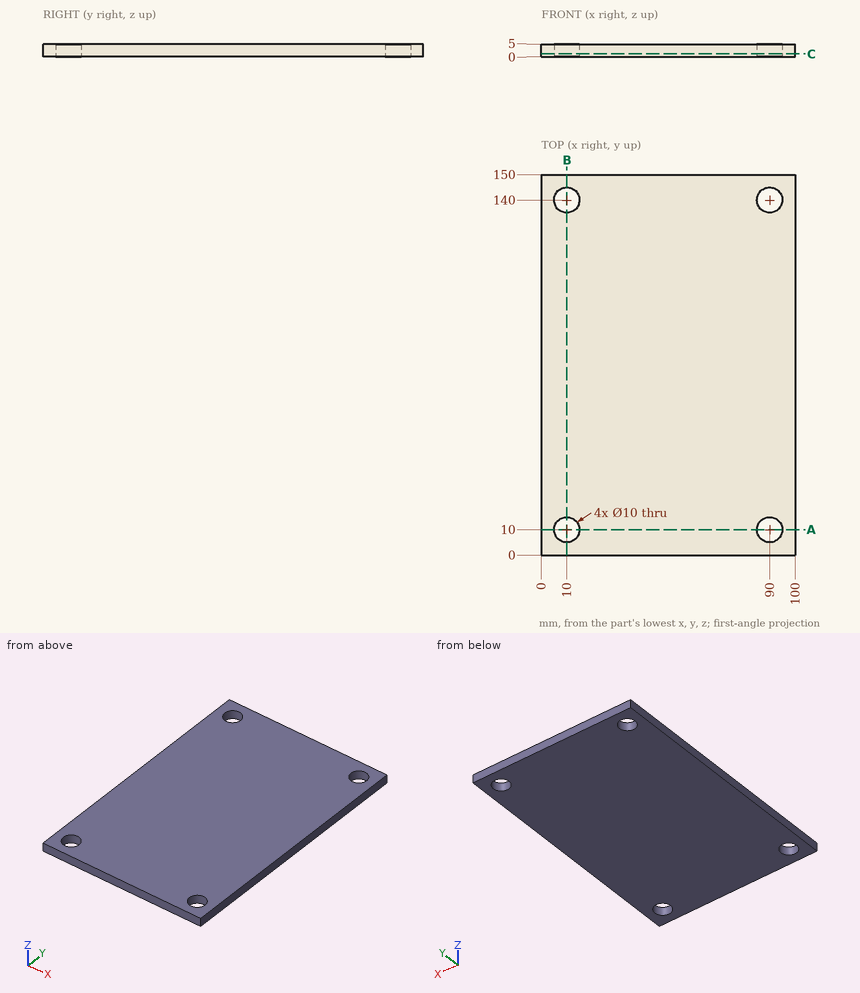
The drawing under review shows one solid part. Ordinate dimensions are in mm from its lowest x, y, z. Give positions to 0.01 mm unless a question says otherwise; leave off trailing zeros. Loops run counter-clockwise (first coordinate to the right, second up) from the corner with the lowest first, then second, coordinate; pieces in that order, holes last. Notation, with made-up numbers: M -0.5,23.25 L 41.5,23.25 A11 cw 41.5,32.25 Z; hole C 12.25,71 d11. An arc over 180 degrees is marked long. Return JSON: item names as keys, results as strings. Group by question number.
Item 1: For probe 1 along Y at (x, z) = (90, 1.4); probe 2 along X at (y, z) = (140, 2.55); probe 3 along X at (y, z) = (143.5, 3), list the stretches that pass through material, from the lowest coordinate up.
Item 2: We need section A-A (y = 10). Give the boundary of the cut face in (x, z).
Item 3: Insertion check: pin 1 Ø8 at (x, y) = (90, 10) entering from +Z. The pin has a flat end and moves straight along its axis. Give the tip position at first contact, or say it passes through.
Item 4: We need section B-B (x = 10). Give the boundary of the cut face in (y, z).
Item 5: We need section C-C (z = 1.1). Give the boundary of the cut face in (x, y), and give its area (3 significant figures).
Output:
{
 "1": {"probe 1": "y = 0 to 5, 15 to 135, 145 to 150", "probe 2": "x = 0 to 5, 15 to 85, 95 to 100", "probe 3": "x = 0 to 6.43, 13.57 to 86.43, 93.57 to 100"},
 "2": {"outline": "M 0,0 L 5,0 L 5,5 L 0,5 Z; M 15,0 L 85,0 L 85,5 L 15,5 Z; M 95,0 L 100,0 L 100,5 L 95,5 Z"},
 "3": {"pin 1": "passes through"},
 "4": {"outline": "M 0,0 L 5,0 L 5,5 L 0,5 Z; M 15,0 L 135,0 L 135,5 L 15,5 Z; M 145,0 L 150,0 L 150,5 L 145,5 Z"},
 "5": {"outline": "M 0,0 L 100,0 L 100,150 L 0,150 Z; hole C 10,10 d10; hole C 10,140 d10; hole C 90,10 d10; hole C 90,140 d10", "area": "14,700 mm^2"}
}
